The listing builds one solid part. Answer for the finished solid, in the listing's coordinates (mm). A direction names the side the tool comes from. Coordinates: 2 decimals unless noted, no trailing zeros. Loops run counter-clockwise (first coordinate to the right, second up) from the corner with the lowest first, then second, coordinate; pieces in that order, holes last. Notation, with made-up numbers: M 27.25,38.5 L 68.25,38.5 A18 ccw 68.25,49.5 Z; hole C -3.5,85 d10. An arc over 180 degrees is marked long. Answer in a Markdown table with one row per item. Add a question column.
from build123d import *

# Parameters (mm, degrees)
BOSS_EXTRUDE1_DEPTH      = 10
CUT_EXTRUDE9_REACH       = 28.107
SKETCH11_R               = 1
CUT_EXTRUDE16_DEPTH      = 14.1
CUT_EXTRUDE16_DEPTH_BACK = 14.1


with BuildPart() as part:
    # Sketch1 → Boss-Extrude1 (new body)
    with BuildSketch(Plane.XY):
        with BuildLine():
            Line((-8.1, 0), (8.1, 0))
            Line((8.1, 0), (8.1, 19.7))
            Line((8.1, 19.7), (8.1, 20.376450886))
            add(Edge.make_bspline(
                [(6.48935173, 24), (7.416747291, 23.101820665), (8.022787745, 21.902680364), (8.1, 20.376450886)],
                knots=[0.795779931, 0.795779931, 0.795779931, 0.795779931, 0.974400134, 0.974400134, 0.974400134, 0.974400134], degree=3))
            Line((6.48935173, 24), (-5.856909443, 24))
            add(Edge.make_bspline(
                [(-8.1, 19.7), (-7.879513959, 21.531569286), (-7.049405333, 22.960789218), (-5.856909443, 24)],
                knots=[0, 0, 0, 0, 0.215700958, 0.215700958, 0.215700958, 0.215700958], degree=3))
            Line((-8.1, 19.7), (-8.1, 0))
        make_face()
        with BuildLine():
            add(Edge.make_bspline(
                [(-5.856909443, 24), (-4.327036412, 25.333220988), (0.13018942, 26.782367162), (4.914346008, 25.525387495), (6.48935173, 24)],
                knots=[0.215700958, 0.215700958, 0.215700958, 0.215700958, 0.492427344, 0.795779931, 0.795779931, 0.795779931, 0.795779931], degree=3))
            Line((-5.856909443, 24), (6.48935173, 24))
        make_face()
    extrude(amount=BOSS_EXTRUDE1_DEPTH)

    # Sketch11 → Cut-Extrude9 (cut, up to next)
    with BuildSketch(Plane.XZ, mode=Mode.PRIVATE) as cut_extrude9_sk1:
        with Locations((4, 2.295920755)):
            Circle(SKETCH11_R)
    cut_extrude9_tool1 = extrude(cut_extrude9_sk1.sketch, amount=-CUT_EXTRUDE9_REACH, mode=Mode.PRIVATE) & part.part
    add(cut_extrude9_tool1.solids().sort_by_distance((4, 0, 2.295921))[0], mode=Mode.SUBTRACT)
    # Sketch11 → Cut-Extrude9 (cut, up to next)
    with BuildSketch(Plane.XZ, mode=Mode.PRIVATE) as cut_extrude9_sk2:
        with Locations((-4, 2.295920755)):
            Circle(SKETCH11_R)
    cut_extrude9_tool2 = extrude(cut_extrude9_sk2.sketch, amount=-CUT_EXTRUDE9_REACH, mode=Mode.PRIVATE) & part.part
    add(cut_extrude9_tool2.solids().sort_by_distance((-4, 0, 2.295921))[0], mode=Mode.SUBTRACT)

    # Sketch14 → Cut-Extrude16 (cut, two sides)
    with BuildSketch(Plane.ZY) as cut_extrude16_sk:
        with BuildLine():
            Line((4.95, 1.181346652), (4.95, 0))
            Line((4.95, 0), (7.05, 0))
            Line((7.05, 0), (7.05, 1.181346652))
            ThreePointArc((7.05, 1.181346652), (6, 5.1), (4.95, 1.181346652))
        make_face()
    extrude(amount=CUT_EXTRUDE16_DEPTH, mode=Mode.SUBTRACT)
    extrude(cut_extrude16_sk.sketch, amount=-CUT_EXTRUDE16_DEPTH_BACK, mode=Mode.SUBTRACT)


solid = part.part
(1) A cutting plane is placed at C-C (y = 21.75). State how many separate pieces and enclosed holes the cut face has, plus the area to 3 significant figures.
(2) For faces 1 (the face through (0, 1, 7.05)), 2 (the face through (-8.1, 10, 5)), determine the directions among +Z, -Z, +X, -X, +Y, -Y from which every point of the face is accessible in a straight line to the end or side of a thin tool.
(3) A cutting plane is placed at A-A (y = 3). Give the vertices of the cut face in (x, z).
(4) Each of these flat-tipped pins is pushed along its axis until it touches: pin 1 (2 mm diameter, centred on x = -1.5, z = 1.5, fed in from +Y); pin 2 (3 mm diameter, centred on x = 3.5, z = 3, fed in from +Y); pin 3 (1 mm diameter, centred on x = 4.5, z = 8, fed in from +Y). Where does it stop, or does it pass through?
(5) Straight lines are drawn through the part: line 1 (X direction, y = 16.5, z = 2.25); line 2 (Z direction, x = 1.25, y = 3); line 3 (Z direction, x = -4, y = 8.75). For each, find the intervals that lie inside material, in ascending order.
(6) A cutting plane is placed at B-B (y = 6.5). Give the vertices of the cut face in (x, z).
(7) The mould has two halves that part along Z. Classify faces 3 (the face through (8.1, 10, 5)), 4 (the face through (0, 14, 0)), 5 (the face through (0, 14, 10)), 6 (the face through (0, 1, 4.95)): released by +Z, released by -Z, zero draft, split by the parting line, or undercut.
Solved:
| question | item | result |
|---|---|---|
| 1 | separate pieces | 1 |
| 1 | enclosed holes | 2 |
| 1 | area | 148 mm² |
| 2 | face 1 | +X, -X, -Y |
| 2 | face 2 | +Z, -Z, -X, +Y, -Y |
| 3 | outline | M -8.1,0 L 8.1,0 L 8.1,3.9 L -8.1,3.9 Z; M -8.1,8.1 L 8.1,8.1 L 8.1,10 L -8.1,10 Z; hole C -4,2.3 d2; hole C 4,2.3 d2 |
| 4 | pin 1 | stops at y = 26.07 |
| 4 | pin 2 | stops at y = 26 |
| 4 | pin 3 | stops at y = 25.51 |
| 5 | line 1 | x = -8.1 to -5, -3 to 3, 5 to 8.1 |
| 5 | line 2 | z = 0 to 3.9, 8.1 to 10 |
| 5 | line 3 | z = 0 to 1.3, 3.3 to 10 |
| 6 | outline | M -8.1,0 L 8.1,0 L 8.1,10 L -8.1,10 Z; hole C -4,2.3 d2; hole C 4,2.3 d2 |
| 7 | face 3 | zero draft |
| 7 | face 4 | released by -Z |
| 7 | face 5 | released by +Z |
| 7 | face 6 | undercut |
